Build history of the part. All positions in model axes, mm. Face numbers are marked on the shaded views. A direction names the side the tool comes from. Round coordinates to 2 decimals unless told otherwise and drop trailing zeros. Write each loop counter-clockwise with the first axis right and the second up, starting at its lowest first coordinate (ties: lowest second). Pieces come first, ordered by that corner, then holes. Notation, with made-up numbers: (-31, -2) -> (5, -2) arc R16 cw to (5, 5) -> close; hole circle Ø9 at (52.25, -23). An arc over 180 degrees is marked (long way). One line per question, with ' | ' between items.
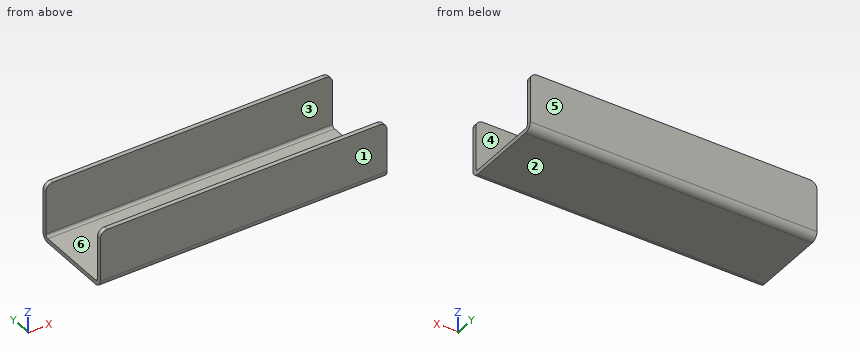
from build123d import *

# Parameters (mm, degrees)
F0_W     = 60
F0_H     = 40
F1_DEPTH = 100
F2_R     = 5
F3_T     = -3
F4_R     = 5


with BuildPart() as f1:
    # F0 (on Right) → F1 (new body, symmetric)
    with BuildSketch(Plane.YZ):
        Rectangle(F0_W, F0_H)
    extrude(amount=F1_DEPTH, both=True)

    # F2
    f2_edges = [f1.edges().sort_by_distance(p)[0] for p in [
        (0, -30, -20),
        (0, 30, -20),
    ]]
    fillet(f2_edges, radius=F2_R)

    # F3
    f3_openings = [f1.faces().sort_by_distance(p)[0] for p in [
        (0, 0, 20),
        (100, 0, 0.084803),
        (-100, 0, 0.084803),
    ]]
    offset(amount=F3_T, openings=f3_openings)

    # F4
    f4_edges = [f1.edges().sort_by_distance(p)[0] for p in [
        (-100, 28.5, 20),
        (-100, -28.5, 20),
        (100, 28.5, 20),
        (100, -28.5, 20),
    ]]
    fillet(f4_edges, radius=F4_R)


solid = f1.part
(1) 3-axis set-ups, long thin cutter, end or side, ignore diameter. For the marked faces 5 and 6: which of +Z, -Z, +X, -X, +Y, -Y reach the whole face in a straight line?
Calculated:
face 5: +Z, -Z, +X, -X, +Y | face 6: +Z, +X, -X
(2) Mould opens along Y. For the marked faces 1, 2, 3 and 4 say: pulls with the +Y half, pulls with the -Y half, needs draft (parallel to the pull), parting line crosses it, or undercut.
Calculated:
face 1: pulls with the -Y half | face 2: needs draft | face 3: undercut | face 4: undercut
(3) Wall check: line 1 (Y direction, x = -47, z = -14); line 2 (Z direction, x = -47, y = -9); line 3 (Z direction, x = -37.5, y = 26.5). Give the ranges that are in metal, low to high. Write a range as from..to.
Calculated:
line 1: -30..-27, 27..30 | line 2: -20..-17 | line 3: -19.77..-16.32
(4) Slice it at A-A (z = -2.5). Write the cut outline in (x, y), then the cut area to 3 significant figures.
Calculated:
outline: (-100, -30) -> (100, -30) -> (100, -27) -> (-100, -27) -> close; (-100, 27) -> (100, 27) -> (100, 30) -> (-100, 30) -> close | area: 1,200 mm2
(5) Drop flat-ended pins along their axis: pin 1 (5 mm diameter, centred on x = -78.5, y = 24, fed in from +Z); pin 2 (12 mm diameter, centred on x = -66, y = -1.5, fed in from +Z). Give the stop position or say it passes through.
Calculated:
pin 1: z = -16.32 | pin 2: z = -17
(6) Slice it at C-C (y = 21.5). Write the cut outline in (x, z), then the cut area to 3 significant figures.
Calculated:
outline: (-100, -20) -> (100, -20) -> (100, -17) -> (-100, -17) -> close | area: 600 mm2
(7) Slice it at B-B (x = 73). Write the cut outline in (y, z), then the cut area to 3 significant figures.
Calculated:
outline: (-30, -15) arc R5 ccw to (-25, -20) -> (25, -20) arc R5 ccw to (30, -15) -> (30, 20) -> (27, 20) -> (27, -15) arc R2 cw to (25, -17) -> (-25, -17) arc R2 cw to (-27, -15) -> (-27, 20) -> (-30, 20) -> close | area: 393 mm2
